Part model, mm, in its own coordinate system. Face numbers are marked on the shaded views. Give positions to 0.01 mm unless a question says otherwise; leave off trailing zeros. Order: outer loops, then holes, each group sorted by start corner. A loop starts at its lowest first (then second) coordinate and runs counter-clockwise, first axis right, second up. Notation, with made-up numbers: (-12.5, 25.25) - (28.5, 25.25) arc R28 ccw to (28.5, 46.25) - close; hole circle Ø8 at (69, 39.5). An arc over 180 degrees is marked (long way). Use one line per item in the form item = value. Start each with the question number.
1. Band-saw the part on B-B, the plane z = 4.75. State how many separate pieces and enclosed holes the cut face has, plus the area to 3 significant figures.
2. Pin check, flat tip, straight feed: P1, Ø2.5, axis at x = 5, y = 21.5, coming from the -Z side. Stop position of the tip, or through.
3. Band-saw the part on D-D, the plane x = 4.75. List the corners of the cut face in (y, z), plus the area to 3 significant figures.
4. Pull direction X, two halves, no side cores. Call the marked faces 1, 2 and 3: +X half, -X half, draft (parallel to the pull), parting line (faces both ways), or undercut.
5. Band-saw the part on A-A, the plane y = 18.5. List the corners of the cut face in (x, z) (3 decimals), plus the area to 3 significant figures.
6. Band-saw the part on C-C, the plane y = 21.5. List the corners of the cut face in (x, z) (3 decimals), plus the area to 3 significant figures.
7. Drill centre lines: line 1 (Y direction, x = 11, z = 1.75) (3 decimals); line 2 (Y direction, x = 4.25, z = 1.75); line 3 (X direction, y = 4, z = 1.5). Where is each one in solid material? Low to high.
from build123d import *

# Parameters (mm, degrees)
SKETCH1_W           = 16
SKETCH1_H           = 25
SKETCH1_R           = 1.325
BOSS_EXTRUDE1_DEPTH = 6.1


with BuildPart() as part:
    # Sketch1 → Boss-Extrude1 (new body)
    with BuildSketch(Plane.XY):
        with Locations((8, 12.5)):
            Rectangle(SKETCH1_W, SKETCH1_H)
        with Locations((2, 12.5)):
            Circle(SKETCH1_R, mode=Mode.SUBTRACT)
        with Locations((8, 18.5)):
            Circle(SKETCH1_R, mode=Mode.SUBTRACT)
        with Locations((5, 21.5)):
            Circle(SKETCH1_R, mode=Mode.SUBTRACT)
        with Locations(Location((14, 12.5, 0), (0, 0, 180))):
            Circle(SKETCH1_R, mode=Mode.SUBTRACT)
        with Locations(Location((11, 21.5, 0), (0, 0, 180))):
            Circle(SKETCH1_R, mode=Mode.SUBTRACT)
        with Locations(Location((5, 3.5, 0), (0, 0, 180))):
            Circle(SKETCH1_R, mode=Mode.SUBTRACT)
        with Locations((11, 3.5)):
            Circle(SKETCH1_R, mode=Mode.SUBTRACT)
        with Locations(Location((8, 6.5, 0), (0, 0, 180))):
            Circle(SKETCH1_R, mode=Mode.SUBTRACT)
    extrude(amount=BOSS_EXTRUDE1_DEPTH)


solid = part.part
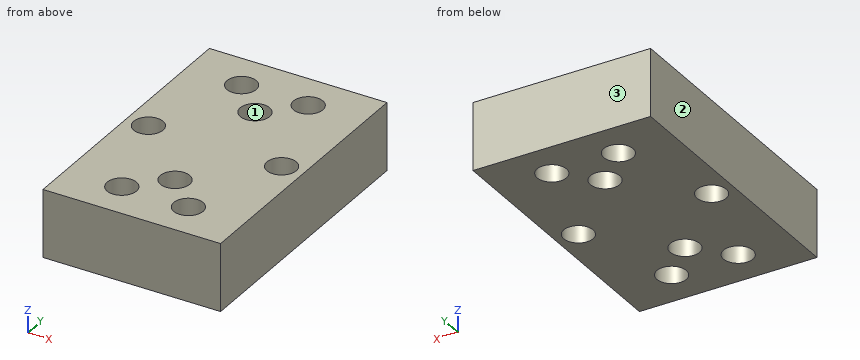
From the geometry:
q1.separate_pieces = 1
q1.enclosed_holes = 8
q1.area = 356 mm²
q2.P1 = through
q3.outline = (0, 0) - (2.2, 0) - (2.2, 6.1) - (0, 6.1) - close; (4.8, 0) - (20.2, 0) - (20.2, 6.1) - (4.8, 6.1) - close; (22.8, 0) - (25, 0) - (25, 6.1) - (22.8, 6.1) - close
q3.area = 121 mm²
q4.face_1 = undercut
q4.face_2 = -X half
q4.face_3 = draft
q5.outline = (0, 0) - (6.675, 0) - (6.675, 6.1) - (0, 6.1) - close; (9.325, 0) - (16, 0) - (16, 6.1) - (9.325, 6.1) - close
q5.area = 81.4 mm²
q6.outline = (0, 0) - (3.675, 0) - (3.675, 6.1) - (0, 6.1) - close; (6.325, 0) - (9.675, 0) - (9.675, 6.1) - (6.325, 6.1) - close; (12.325, 0) - (16, 0) - (16, 6.1) - (12.325, 6.1) - close
q6.area = 65.3 mm²
q7.line_1 = 0 to 2.175, 4.825 to 20.175, 22.825 to 25
q7.line_2 = 0 to 2.41, 4.59 to 20.41, 22.59 to 25
q7.line_3 = 0 to 3.77, 6.23 to 9.77, 12.23 to 16
